```python
from build123d import *

# Parameters (mm, degrees)
F0_W     = 40
F0_H     = 40
F0_W_2   = 13
F0_H_2   = 13
F1_DEPTH = 10
F2_DEPTH = 7
F0_W_3   = 10
F3_DEPTH = 10
F4_R     = 4.99999
F5_R     = 5
F6_D     = 5.5
F6_DEPTH = 7
F6_TIP   = 1.6523667023


# Not quite as in the source:
# - a fillet or chamfer is up to 0.001 mm smaller than in the source, because OpenCascade refuses the exact size
# - a feature names something its author has since deleted; it is built from what else it names


with BuildPart() as f1:
    # F0 (on Front) → F1 (new body)
    with BuildSketch(Plane.XZ):
        Rectangle(F0_W, F0_H)
        Polygon((-18, 3.6852569133), (-18, 16.6852569133), (-5, 16.6852569133), (5, 16.6852569133), (18, 16.6852569133), (18, 3.6852569133), (5, 3.6852569133), (-5, 3.6852569133), align=None, mode=Mode.SUBTRACT)
        with Locations((-11.5, 10.1852569133)):
            Rectangle(F0_W_2, F0_H_2)
        with Locations((11.5, 10.1852569133)):
            Rectangle(F0_W_2, F0_H_2)
    extrude(amount=-F1_DEPTH)

    # F0 (on Front) → F2 (cut)
    with BuildSketch(Plane.XZ):
        with Locations((-11.5, 10.1852569133)):
            Rectangle(F0_W_2, F0_H_2)
        with Locations((11.5, 10.1852569133)):
            Rectangle(F0_W_2, F0_H_2)
    extrude(amount=-F2_DEPTH, mode=Mode.SUBTRACT)

    # F0 (on Front) → F3 (join)
    with BuildSketch(Plane.XZ):
        with Locations((0, 10.1852569133)):
            Rectangle(F0_W_3, F0_H_2)
    extrude(amount=-F3_DEPTH)

    # F4 (radius 5 in the source; OpenCascade refuses exactly that, so slightly less here)
    f4_edges = [f1.edges().sort_by_distance(p)[0] for p in [
        (5, 0, 10.185257),
        (-5, 0, 10.185257),
    ]]
    fillet(f4_edges, radius=F4_R)

    # F5
    f5_edges = [f1.edges().sort_by_distance(p)[0] for p in [
        (0, 10, 20),
        (20, 5, 20),
        (-20, 5, 20),
        (20, 5, -20),
        (0, 10, -20),
        (-20, 5, -20),
        (-20, 10, 0),
        (20, 10, 0),
    ]]
    fillet(f5_edges, radius=F5_R)

    # F6
    with Locations(Plane.XZ):
        with Locations((-10, -10), (10, -10)):
            Hole(F6_D / 2, depth=F6_DEPTH)
            with Locations((0, 0, -(F6_DEPTH + F6_TIP / 2))):  # 118° drill point
                Cone(0, F6_D / 2, F6_TIP, mode=Mode.SUBTRACT)


solid = f1.part
```
Geometry check sheet. Reference: the model listing, model coordinates, mm. A direction names the side the tool comes from. Coordinates: 2 decimals unless noted, no trailing zeros. Loops run counter-clockwise (first coordinate to the right, second up) from the corner with the lowest first, then second, coordinate; pieces in that order, holes last. Notation, with made-up numbers: (32, -12.75) -> (71, -12.75) arc R28 ccw to (71, 25.25) -> close; hole circle Ø10 at (66, 50.5). An arc over 180 degrees is marked (long way). Put each result on its own line as item: value.
1) Cross-section at C-C on x = -13.5. Record the boundary of the cut face in (y, z), plus the area to 3 significant figures.
Result set:
outline: (0, -20) -> (5, -20) arc R5 ccw to (10, -15) -> (10, 15) arc R5 ccw to (5, 20) -> (0, 20) -> (0, 16.69) -> (7, 16.69) -> (7, 3.69) -> (0, 3.69) -> close
area: 298 mm^2
2) Cross-section at D-D on z = -1. Record the boundary of the cut face in (x, y).
Result set:
outline: (-20, 0) -> (20, 0) -> (20, 5) arc R5 ccw to (15, 10) -> (-15, 10) arc R5 ccw to (-20, 5) -> close
3) Tool access check on faces 4 (the flat face through (-18, 3, 10)), 5 (the cylindrical face through (0, 8, 19)). Record the directions out of +Z, -Z, +X, -X, +Y, -Y that give a thin tool (end or side, any length) a straight path to the whole face; none if there is none.
Result set:
face 4: -Y
face 5: +Z, +X, -X, +Y
4) Release check for a two-part mould opening along X. For faces 1 (the cylindrical face through (0, 9, -18)), 2 (the cylindrical face through (-12.62, 3.55, -9.17)), 3 (the cylindrical face through (18, 9, 0)) record: released by +X, released by -X, zero draft, split by the parting line, or undercut.
Result set:
face 1: zero draft
face 2: undercut
face 3: released by +X
5) Gauge pin test, flat ends, axial feed: pin 1 Ø10 at (x, z) = (6, 10.5) entering from -Y; pin 2 Ø1.6 at (y, z) = (6, 13.5) entering from +X; pin 3 Ø0.6 at (y, z) = (6.5, 10.5) entering from -X. Record the tip position at first contact, or that the pin passes through.
Result set:
pin 1: stops at y = 0.1
pin 2: stops at x = 20
pin 3: stops at x = -19.85
6) Thickness scan on line 1 (Z direction, x = -10, y = 4.25); line 2 (X direction, y = 5.25, z = -10); line 3 (Z direction, x = 14, y = 0.5). Record the ranges inside material, lowest first.
Result set:
line 1: z = -20 to -12.75, -7.25 to 3.69, 16.69 to 20
line 2: x = -19.99 to -12.75, -7.25 to 7.25, 12.75 to 19.99
line 3: z = -20 to 3.69, 16.69 to 20
7) Cross-section at B-B on y = 5.75. Record the boundary of the cut face in (x, z), plus the area to 3 significant figures.
Result set:
outline: (-19.94, -15) arc R4.94 ccw to (-15, -19.94) -> (15, -19.94) arc R4.94 ccw to (19.94, -15) -> (19.94, 15) arc R4.94 ccw to (15, 19.94) -> (-15, 19.94) arc R4.94 ccw to (-19.94, 15) -> close; hole (-18, 3.69) -> (-5, 3.69) -> (-5, 16.69) -> (-18, 16.69) -> close; hole circle Ø5.5 at (-10, -10); hole (5, 3.69) -> (18, 3.69) -> (18, 16.69) -> (5, 16.69) -> close; hole circle Ø5.5 at (10, -10)
area: 1,180 mm^2
